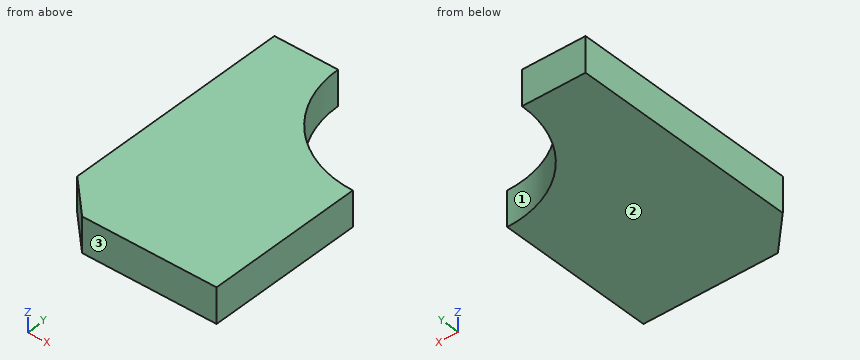
from build123d import *

# Parameters (mm, degrees)
SKETCH_W     = 48.25
SKETCH_H     = 75.15
PAD_DEPTH    = 10
SKETCH001_R  = 30.15
POCKET_DEPTH = 10.001


with BuildPart() as part:
    # Sketch → Pad (new body)
    with BuildSketch(Plane.XY):
        with Locations((24.125, 37.575)):
            Rectangle(SKETCH_W, SKETCH_H)
    extrude(amount=PAD_DEPTH)

    # Sketch001 (on Face6 of Pad) → Pocket (cut, through all)
    with BuildSketch(Plane.XY.offset(10)):
        with Locations((48.25, 75.15)):
            Circle(SKETCH001_R)
        Polygon((0, 10), (10, 0), (0, 0), align=None)
    extrude(amount=-POCKET_DEPTH, mode=Mode.SUBTRACT)


solid = part.part
For this review, take the finished solid that the model builds, in its own axes (mm). Face numbers are marked on the shaded views. Coordinates: 2 decimals unless noted, no trailing zeros. Order: outer loops, then holes, each group sorted by start corner. A loop starts at its lowest first (then second) coordinate and runs counter-clockwise, first axis right, second up. Notation, with made-up numbers: (79.5, 80.25) - (133.5, 80.25) arc R12 ccw to (133.5, 92.25) - close; hole circle Ø1 at (48.5, -10). An arc over 180 degrees is marked (long way). Use one line per item in the form item = value.
Q1. Consider section B-B (x = 5). Give the boundary of the cut face in (y, z), then the cut area to 4 significant figures.
Checked values:
outline = (5, 0) - (75.15, 0) - (75.15, 10) - (5, 10) - close
area = 701.5 mm2
Q2. For probe 1 along X at (y, z) = (70.5, 7.75); probe 2 along Y at (x, z) = (40, 8); probe 3 along Y at (x, z) = (7.5, 9.75), list the stretches that pass through material, from the lowest coordinate up. Write a range as from..to.
Checked values:
probe_1 = 0..18.46
probe_2 = 0..46.15
probe_3 = 2.5..75.15
Q3. For P1, Ø1, axis at y = 54, z = 6, coming from the +X side, flat-tipped, find the tip position at first contact; note if it passes through.
Checked values:
P1 = 27.27
Q4. Consider section A-A (z = 6.25). Give the boundary of the cut face in (x, y), then the cut area to 3 significant figures.
Checked values:
outline = (0, 10) - (10, 0) - (48.25, 0) - (48.25, 45) arc R30.15 cw to (18.1, 75.15) - (0, 75.15) - close
area = 2,860 mm2
Q5. Draft analysis for pull direction Y (two halves, no side actions). For the marked faces 1, 2 and 3, state which applies: +Y half, -Y half, draft (parallel to the pull), parting line (faces both ways), or undercut.
Checked values:
face_1 = +Y half
face_2 = draft
face_3 = -Y half
Q6. Consider section C-C (y = 49.5). Give the boundary of the cut face in (x, z).
Checked values:
outline = (0, 0) - (32.4, 0) - (32.4, 10) - (0, 10) - close
